```python
from build123d import *

# Parameters (mm, degrees)
SKETCH1_R           = 2.95
BOSS_EXTRUDE1_DEPTH = 1
SKETCH2_R           = 2.5
BOSS_EXTRUDE2_DEPTH = 7.6
CUT_EXTRUDE1_START  = -7.6
CUT_EXTRUDE1_DEPTH  = 7.6
FILLET1_R           = 2.5
SKETCH4_W           = 0.5
SKETCH4_H           = 0.5
BOSS_EXTRUDE3_DEPTH = 3


with BuildPart() as part:
    # Sketch1 → Boss-Extrude1 (new body)
    with BuildSketch(Plane(origin=(0, 0, 0), x_dir=(1, 0, 0), z_dir=(0, 1, 0))):
        with Locations(Location((0, 0, 0), (0, 0, 270))):
            Circle(SKETCH1_R)
    extrude(amount=BOSS_EXTRUDE1_DEPTH)

    # Sketch2 → Boss-Extrude2 (add)
    with BuildSketch(Plane(origin=(0, 1, 0), x_dir=(1, 0, 0), z_dir=(0, 1, 0))):
        with Locations(Location((0, 0, 0), (0, 0, 90))):
            Circle(SKETCH2_R)
    extrude(amount=BOSS_EXTRUDE2_DEPTH)

    # Sketch3 → Cut-Extrude1 (cut)
    with BuildSketch(Plane(origin=(0, 1, 0), x_dir=(1, 0, 0), z_dir=(0, 1, 0)).offset(CUT_EXTRUDE1_START)):
        with BuildLine():
            Line((-1.566045976, 2.5), (1.566045976, 2.5))
            ThreePointArc((1.566045976, 2.5), (0, 2.95), (-1.566045976, 2.5))
        make_face()
    extrude(amount=CUT_EXTRUDE1_DEPTH, mode=Mode.SUBTRACT)

    # Fillet1
    fillet1_edges = [part.edges().sort_by_distance(p)[0] for p in [
        (0, 8.6, 2.5),
    ]]
    fillet(fillet1_edges, radius=FILLET1_R)

    # Sketch4 → Boss-Extrude3 (add)
    with BuildSketch(Plane.XZ):
        with Locations((0, 1.27)):
            Rectangle(SKETCH4_W, SKETCH4_H)
        with Locations((0, -1.27)):
            Rectangle(SKETCH4_W, SKETCH4_H)
    extrude(amount=BOSS_EXTRUDE3_DEPTH)


solid = part.part
```
CAD build for the part. Positions are in the model's coordinates, mm. A direction names the side the tool comes from. Coordinates: 2 decimals unless noted, no trailing zeros. Write each loop counter-clockwise with the first axis right and the second up, starting at its lowest first coordinate (ties: lowest second). Pieces come first, ordered by that corner, then holes.
(1) Cut at B-B, the plane z = 0. List the corners of the cut face in (x, y).
(2) Flat gauge pins, fed straight in: pin 1 (1.5 mm diameter, centred on x = -2, y = 7.5, fed in from -Z); pin 2 (2 mm diameter, centred on x = 2, y = 7, fed in from -Z); pin 3 (1.6 mm diameter, centred on x = 1, z = 0, fed in from +Y). Where does each tip first touch, or does it go through?
(3) Cut at C-C, the plane x = 1.35. List the corners of the cut face in (y, z).
(4) 3-axis set-ups, long thin cutter, end or side, ignore diameter. For faces 1 (the face through (2.44, 3.51, 0.54)), 2 (the face through (-0.107, 0.493, 2.948)): which of +Z, -Z, +X, -X, +Y, -Y reach the whole face in a straight line?
(5) Cut at D-D, the plane y = 4.75. List the corners of the cut face in (x, z).
(6) Cut at A-A, the plane y = -2. List the corners of the cut face in (x, z).
(7) Drill centre lines: probe 1 along Y at (x, z) = (-2.2, 1.65); probe 2 along X at (y, z) = (2.25, 0); probe 3 along X at (y, z) = (6.25, -0.65). Where is each one in solid material? Low to high.
Geometry says:
1. outline: (-2.95, 0) - (2.95, 0) - (2.95, 1) - (2.5, 1) - (2.5, 6.1) arc R2.5 ccw to (-2.5, 6.1) - (-2.5, 1) - (-2.95, 1) - close
2. pin 1: stops at z = -1.84
2. pin 2: stops at z = -2.2
2. pin 3: stops at y = 8.59
3. outline: (0, -2.5) - (1, -2.5) - (1, -2.1) - (6.1, -2.1) arc R2.1 ccw to (6.1, 2.1) - (1, 2.1) - (1, 2.62) - (0, 2.62) - close
4. face 1: +Y
4. face 2: +Y, -Y
5. outline: circle Ø5 at (0, 0)
6. outline: (-0.25, -1.52) - (0.25, -1.52) - (0.25, -1.02) - (-0.25, -1.02) - close; (-0.25, 1.02) - (0.25, 1.02) - (0.25, 1.52) - (-0.25, 1.52) - close
7. probe 1: y = 0 to 1
7. probe 2: x = -2.5 to 2.5
7. probe 3: x = -2.41 to 2.41
